from build123d import *

# Parameters (mm, degrees)
F1_DEPTH = 11
F2_D     = 6.5
F3_DEPTH = 38.9


with BuildPart() as f1:
    # F0 (on Top) → F1 (new body)
    with BuildSketch(Plane.XY):
        with BuildLine():
            Line((-37.3461883515, 23.3051764891), (-37.3461883515, -25.6948235109))
            Line((-37.3461883515, -25.6948235109), (37.6538116485, -25.6948235109))
            Line((37.6538116485, -25.6948235109), (37.6538116485, 23.3051764891))
            Line((37.6538116485, 23.3051764891), (21.6870121658, 23.3051764891))
            add(Edge.make_bspline(
                [(-18.8461883515, 23.3051764891), (-13.3813479915, 10.3051764891), (-1.0917122471, 10.3051764891), (17.0727558434, 10.3051764891), (21.6870121658, 23.3051764891)],
                knots=[0, 0, 0, 0, 0.4875911488, 1, 1, 1, 1], degree=3))
            Line((-18.8461883515, 23.3051764891), (-37.3461883515, 23.3051764891))
        make_face()
        with BuildLine():
            Line((21.6870121658, 23.3051764891), (-18.8461883515, 23.3051764891))
            add(Edge.make_bspline(
                [(-18.8461883515, 23.3051764891), (-13.3813479915, 10.3051764891), (-1.0917122471, 10.3051764891), (17.0727558434, 10.3051764891), (21.6870121658, 23.3051764891)],
                knots=[0, 0, 0, 0, 0.4875911488, 1, 1, 1, 1], degree=3))
        make_face()
    extrude(amount=F1_DEPTH)

    # F2 (through all)
    with Locations(Plane(origin=(0, 0, 0), x_dir=(1, 0, 0), z_dir=(0, 0, -1))):
        with Locations((19.1538116485, -10.3051764891), (-18.8461883515, -10.3051764891)):
            Hole(F2_D / 2)

    # F0 (on Top) → F3 (cut)
    with BuildSketch(Plane.XY):
        with BuildLine():
            Line((21.6870121658, 23.3051764891), (-18.8461883515, 23.3051764891))
            add(Edge.make_bspline(
                [(-18.8461883515, 23.3051764891), (-13.3813479915, 10.3051764891), (-1.0917122471, 10.3051764891), (17.0727558434, 10.3051764891), (21.6870121658, 23.3051764891)],
                knots=[0, 0, 0, 0, 0.4875911488, 1, 1, 1, 1], degree=3))
        make_face()
    extrude(amount=F3_DEPTH, mode=Mode.SUBTRACT)


solid = f1.part
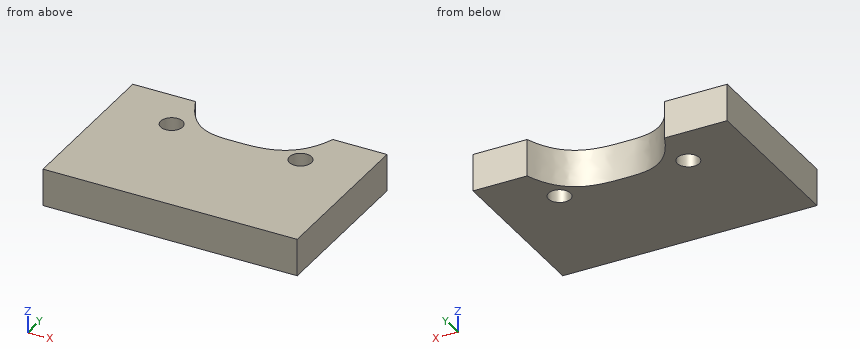
Geometry check sheet. Reference: the model listing, model coordinates, mm. Give positions to 0.01 mm unless a question says otherwise; leave off trailing zeros. Order: outer loops, then holes, each group sorted by start corner. A loop starts at its lowest first (then second) coordinate and runs counter-clockwise, first axis right, second up. Notation, with made-up numbers: M 87.25,67.5 L 119.25,67.5 A24 ccw 119.25,77.5 Z; hole C 71,42.25 d6. An arc over 180 degrees is marked long. Use a Markdown table: item, result.
Item 1: Section check C-C (z = 9). State how many separate pieces and enclosed holes the cut face has, and give its area (3 significant figures).
Answers follow:
| item | result |
|---|---|
| separate pieces | 1 |
| enclosed holes | 2 |
| area | 3,200 mm2 |
Item 2: Material ranges on line 1 along Y through (x, z) = (-19, 2); line 2 along Y through (x, z) = (21, 2.5); line 3 along X through (y, z) = (21, 3.5), recorded low to high.
Answers follow:
| item | result |
|---|---|
| line 1 | y = -25.69 to 7.06, 13.55 to 23.31 |
| line 2 | y = -25.69 to 7.63, 12.98 to 21.54 |
| line 3 | x = -37.35 to -17.81, 20.76 to 37.65 |
Item 3: Depth check by flat-ended pin: P1, Ø6, axis at x = -2, z = 1.5, coming from the +Y side; P2, Ø5, axis at x = -9, z = 5.5, coming from the +Y side. Enter the tip coordinate at first touch or a pass-through.
Answers follow:
| item | result |
|---|---|
| P1 | stops at y = 10.48 |
| P2 | stops at y = 12.76 |
Item 4: Section check A-A (y = 9.5). Record the cut outline in (x, z).
Answers follow:
| item | result |
|---|---|
| outline | M -37.35,0 L -21.99,0 L -21.99,11 L -37.35,11 Z; M -15.7,0 L 16.01,0 L 16.01,11 L -15.7,11 Z; M 22.3,0 L 37.65,0 L 37.65,11 L 22.3,11 Z |
Item 5: Section check B-B (x = -20.5). Record the cut outline in (y, z).
Answers follow:
| item | result |
|---|---|
| outline | M -25.69,0 L 7.51,0 L 7.51,11 L -25.69,11 Z; M 13.1,0 L 23.31,0 L 23.31,11 L 13.1,11 Z |
